Source: CAD feature listing. Evaluate the final solid. Frame: model axes, mm. A direction names the side the tool comes from. Give positions to 0.01 mm unless a question says otherwise; leave off trailing zeros. Write each loop counter-clockwise with the first axis right and the second up, starting at its lowest first coordinate (ties: lowest second). Pieces come first, ordered by that corner, then holes. Notation, with made-up numbers: M 58,73.25 L 76,73.25 A26 cw 76,100.25 Z; hole C -15,-23.75 d11. An arc over 180 degrees is marked long. Return JSON: item names as keys, results as strings.
Autodesk Inventor part; units mm, degrees
ref_plane "YZ Plane" through (0, 0, 0) normal (1, 0, 0) x (0, 1, 0)
ref_plane "XZ Plane" through (0, 0, 0) normal (0, 1, 0) x (-1, 0, 0)
ref_plane "XY Plane" through (0, 0, 0) normal (0, 0, 1) x (1, 0, 0)
sketch "Sketch1" plane through (0, 0, 0) normal (0, 0, 1) x (1, 0, 0)
  line L0 (0, 0) -> (60, 0)
  line L1 (60, 0) -> (60, 60)
  line L2 (60, 60) -> (0, 60)
  line L3 (0, 60) -> (0, 0)
  dimension "d0" = 60
  dimension "d1" = 60
extrude "Extrusion1" add sketch "Sketch1" along normal blind 5
sketch "Sketch2" plane through (0, 0, 5) normal (0, 0, 1) x (1, 0, 0)
  line L0 (60, 60) -> (0, 60)
  line L1 (60, 0) -> (60, 60)
  point P0 (0, 0)
  point P1 (30, 30)
  dimension "d4" = 30
  dimension "d5" = 30
hole "Hole1" at (30, 30, 5) direction (0, 0, -1) diameter 15 end through all
fillet "Fillet1" radius 2 4 edges at (60, 60, 2.5) (60, 0, 2.5) (0, 0, 2.5) (0, 60, 2.5)
sketch "Sketch5" plane through (0, 2, 0) normal (-1, 0, 0) x (0, 0, 1)
  line L0 (0, 56) -> (0, 0)
  line L1 (0, -2) -> (5, -2)
  point P0 (2.5, 33)
  dimension "d36" = 2.5
  dimension "d37" = 35
hole "Hole4" at (0, 35, 2.5) direction (1, 0, 0) diameter 2 depth 10 tip angle 118
properties part number "Motor clamp p1"
1) Cut plane B-B, the plane z = 4.3. Return the cut outline in (x, y).
Numbers:
{"outline": "M 0,2 A2 ccw 2,0 L 58,0 A2 ccw 60,2 L 60,58 A2 ccw 58,60 L 2,60 A2 ccw 0,58 Z; hole C 30,30 d15"}
2) Cut plane A-A, the plane y = 30. Return the cut outline in (x, z).
Numbers:
{"outline": "M 0,0 L 22.5,0 L 22.5,5 L 0,5 Z; M 37.5,0 L 60,0 L 60,5 L 37.5,5 Z"}
3) Line query: line 1 (Y direction, x = 30, z = 3.3); line 2 (Y direction, x = 6.25, z = 2.5). Output: solid intervals per line, ascending. Write a range as [from, to].
Numbers:
{"line 1": "y = [0, 22.5], [37.5, 60]", "line 2": "y = [0, 34], [36, 60]"}
4) Draft query along Z for faces 3 (the face through (10.497, 35.146, 2.593)), 4 (the face through (23, 24, 5)), 5 (the face through (0, 30, 2)), 6 (the face through (23, 24, 0)). Return one class per face: released by +Z, released by -Z, zero draft, split by the parting line, or undercut.
Numbers:
{"face 3": "undercut", "face 4": "released by +Z", "face 5": "zero draft", "face 6": "released by -Z"}
5) Set-up query: faces 1 (the face through (30, 0, 2)), 2 (the face through (5.07, 34.01, 2.37)). Return all of +Z, -Z, +X, -X, +Y, -Y with unobstructed straight access to the full face (end or side cutting, diameter ignored); none if empty.
Numbers:
{"face 1": "+Z, -Z, +X, -X, -Y", "face 2": "-X"}
